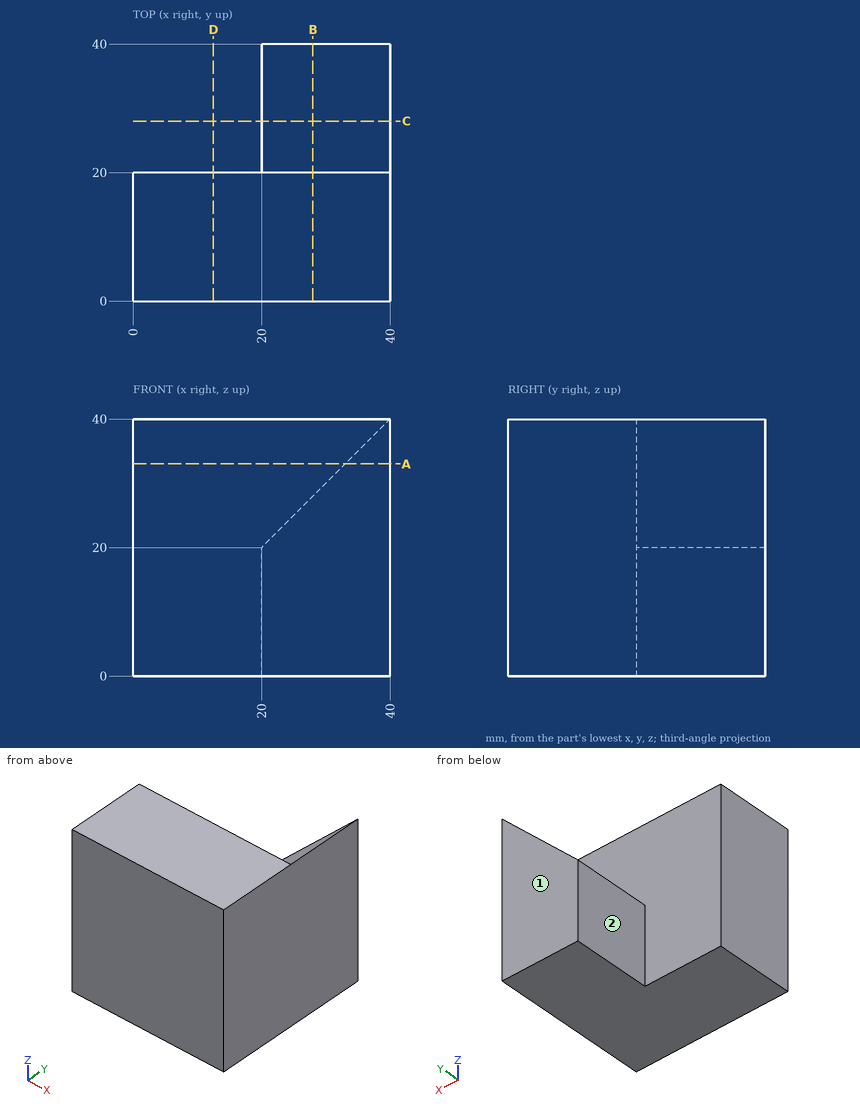
Verification items for this drawing (mm, ordinates from the low corner). A direction names the side the tool comes from. Coordinates: 2 decimals unless noted, no trailing zeros. Write each loop counter-clockwise with the first axis right and the second up, starting at its lowest first coordinate (ties: lowest second). Pieces come first, ordered by that corner, then holes. Notation, with made-up numbers: M -20.75,70 L 25.25,70 A15 ccw 25.25,88 Z; hole C 47,74 d9. An arc over 180 degrees is marked long. Use CSV: the item, a comma, the result in double quotes.
Q1. Section check D-D, the plane x = 12.5. Enter the section's corners in (y, z).
Computed values:
outline,"M 0,0 L 20,0 L 20,40 L 0,40 Z"
Q2. Section check A-A, the plane z = 33. Enter the section's corners in (x, y), and give its area (3 significant figures).
Computed values:
outline,"M 0,0 L 40,0 L 40,40 L 33,40 L 33,20 L 0,20 Z"
area,"940 mm²"
Q3. Set-up check for the marked faces 1 and 2: record each of +Z, -Z, +X, -X, +Y, -Y from which the full face is reachable in a straight line by a thin tool's end or side.
Computed values:
face 1,"+Z, -Z, +X, -X, +Y"
face 2,"+Z, -Z, -X, +Y"
Q4. Section check C-C, the plane y = 28. Enter the section's corners in (x, z).
Computed values:
outline,"M 20,0 L 40,0 L 40,40 L 20,20 Z"
Q5. Thickness scan on line 1 along Y through (x, z) = (4, 22); line 2 along X through (y, z) = (36.5, 5); line 3 along Z through (x, y) = (37.5, 34). Record the ranges inside material, lowest first. Write a range as [from, to].
Computed values:
line 1,"[0, 20]"
line 2,"[20, 40]"
line 3,"[0, 37.5]"
Q6. Go/stop test with flat-tipped pins: P1, Ø5, axis at x = 9.5, z = 12.5, coming from the +Y side; P2, Ø16, axis at y = 31.5, z = 7, coming from the -X side. Record where each tip stops, or that it passes through.
Computed values:
P1,"y = 20"
P2,"x = 20"
Q7. Section check B-B, the plane x = 28. Enter the section's corners in (y, z), and give its area (3 significant figures).
Computed values:
outline,"M 0,0 L 40,0 L 40,28 L 20,28 L 20,40 L 0,40 Z"
area,"1,360 mm²"
